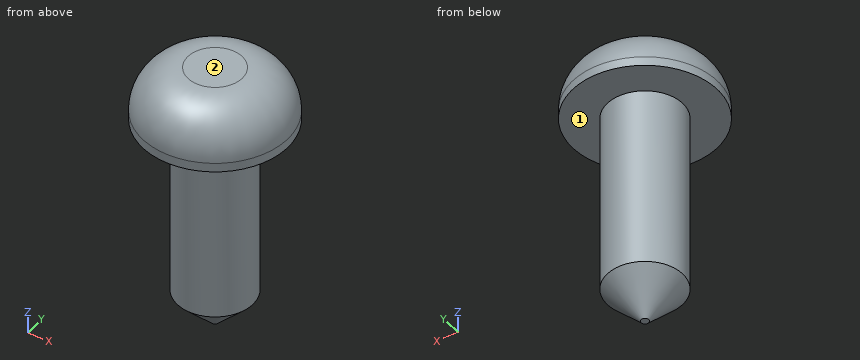
from build123d import *

# Parameters (mm, degrees)
SKETCH1_R           = 4.064
BOSS_EXTRUDE1_DEPTH = 3.048
SKETCH2_R           = 2.1209
BOSS_EXTRUDE2_DEPTH = 12.065
CHAMFER1_SIZE       = 1.905
FILLET1_R           = 2.54


with BuildPart() as part:
    # Sketch1 → Boss-Extrude1 (new body)
    with BuildSketch(Plane.XY):
        Circle(SKETCH1_R)
    extrude(amount=BOSS_EXTRUDE1_DEPTH)

    # Sketch2 → Boss-Extrude2 (add)
    with BuildSketch(Plane(origin=(0, 0, 0), x_dir=(-1, 0, 0), z_dir=(0, 0, -1))):
        Circle(SKETCH2_R)
    extrude(amount=BOSS_EXTRUDE2_DEPTH)

    # Chamfer1
    chamfer1_edges = [part.edges().sort_by_distance(p)[0] for p in [
        (2.1209, 0, -12.065),
    ]]
    chamfer(chamfer1_edges, length=CHAMFER1_SIZE)

    # Fillet1
    fillet1_edges = [part.edges().sort_by_distance(p)[0] for p in [
        (-4.064, 0, 3.048),
    ]]
    fillet(fillet1_edges, radius=FILLET1_R)


solid = part.part
CAD build for the part. Positions are in the model's coordinates, mm. Face numbers are marked on the shaded views. A direction names the side the tool comes from. Round coordinates to 2 decimals unless told otherwise and drop trailing zeros. Order: outer loops, then holes, each group sorted by start corner. A loop starts at its lowest first (then second) coordinate and runs counter-clockwise, first axis right, second up. Notation, with made-up numbers: (25.25, 4.5) - (66.25, 4.5) arc R18 cw to (66.25, 11.5) - close; hole circle Ø8 at (-37.75, 36). An arc over 180 degrees is marked (long way). Return JSON: item names as keys, results as strings.
(1) Cut at A-A (z = -2.25). Give the cut face in (x, y).
Answer key:
{"outline": "circle Ø4.24 at (0, 0)"}
(2) Tool access for the marked faces 1 and 2: list every direction of +Z, -Z, +X, -X, +Y, -Y with a clear straight run to the whole face (end or side of a thin tool).
Answer key:
{"face 1": "-Z", "face 2": "+Z, +X, -X, +Y, -Y"}
(3) Wall check: probe 1 along Y at (x, z) = (0.25, -2); probe 2 along X at (y, z) = (-1.5, -6.75); probe 3 along Z at (x, y) = (-1, 2). Give the ranges that are in metal, low to high. Write a range as from..to.
Answer key:
{"probe 1": "y = -2.11..2.11", "probe 2": "x = -1.5..1.5", "probe 3": "z = 0..2.95"}
(4) Pin check, flat tips, straight feed: pin 1 Ø4 at (y, z) = (1.5, -9) entering from +X; pin 2 Ø3 at (x, z) = (-3, -4.5) entering from +Y; pin 3 Ø1 at (x, y) = (1.5, -2) entering from -Z. Stop position of each tip, or through.
Answer key:
{"pin 1": "stops at x = 2.12", "pin 2": "stops at y = 1.5", "pin 3": "stops at z = -10.28"}
